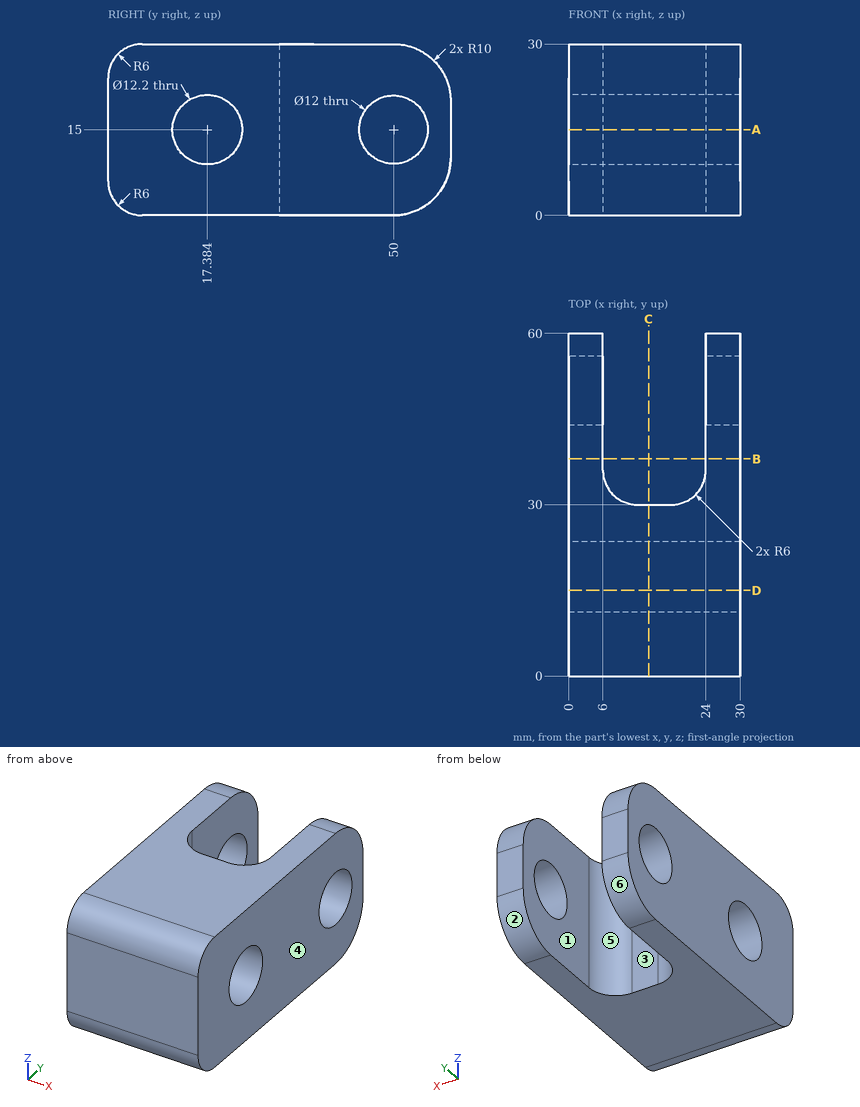
Answer from the drawing. Dimensions are ordinates in mm from the lowest x, y and z of the part. A direction names the side the tool comes from. Coordinates: 2 decimals unless noted, no trailing zeros. Loops run counter-clockwise (first coordinate to the right, second up) from the corner with the lowest first, then second, coordinate; pieces in that order, holes last. Notation, with made-up numbers: (-22, 42) -> (35, 42) arc R18 ccw to (35, 46) -> close; hole circle Ø1 at (-16.75, 8.5). An arc over 180 degrees is marked (long way). Return JSON: item names as keys, results as strings.
Item 1: Find section C-C (x = 14). Determine the outline of the cut face in (y, z).
Answers:
{"outline": "(0, 6) arc R6 ccw to (6, 0) -> (30, 0) -> (30, 30) -> (6, 30) arc R6 ccw to (0, 24) -> close; hole circle Ø12.2 at (17.38, 15)"}
Item 2: For the marked faces 1 and 2, determine the directions among +Z, -Z, +X, -X, +Y, -Y from which every point of the face is accessible in a straight line to the end or side of a thin tool.
Answers:
{"face 1": "+Z, -Z, +Y", "face 2": "-Z, +X, -X, +Y"}
Item 3: Find section D-D (y = 15). Determine the outline of the cut face in (x, z) (1 decimal).
Answers:
{"outline": "(0, 0) -> (30, 0) -> (30, 9.4) -> (0, 9.4) -> close; (0, 20.6) -> (30, 20.6) -> (30, 30) -> (0, 30) -> close"}
Item 4: Find section B-B (y = 38). Determine the outline of the cut face in (x, z), plus the area to 3 significant figures.
Answers:
{"outline": "(0, 0) -> (6, 0) -> (6, 30) -> (0, 30) -> close; (24, 0) -> (30, 0) -> (30, 30) -> (24, 30) -> close", "area": "360 mm2"}
Item 5: Find section A-A (z = 15). Determine the outline of the cut face in (x, y).
Answers:
{"outline": "(0, 0) -> (30, 0) -> (30, 11.28) -> (0, 11.28) -> close; (0, 23.48) -> (30, 23.48) -> (30, 44) -> (24, 44) -> (24, 36) arc R6 cw to (18, 30) -> (12, 30) arc R6 cw to (6, 36) -> (6, 44) -> (0, 44) -> close; (0, 56) -> (6, 56) -> (6, 60) -> (0, 60) -> close; (24, 56) -> (30, 56) -> (30, 60) -> (24, 60) -> close"}
Item 6: Flat-ended cylindrical pins translate along their axes: P1, Ø7, axis at y = 50, z = 15, coming from the -X side; P2, Ø6.5, axis at x = 15.5, z = 16, coming from the +Y side. Find the tip coordinate at first contact, or state that the pin passes through.
Answers:
{"P1": "passes through", "P2": "stops at y = 30.05"}
Item 7: For a pull along X with two mould halves and no side action, classify the marked faces 3, 4, 5 and 6 as +X half, -X half, draft (parallel to the pull), parting line (faces both ways), or undercut.
Answers:
{"face 3": "undercut", "face 4": "+X half", "face 5": "undercut", "face 6": "draft"}
Item 8: Find the intervals of material crossed by probe 1 along Z at (x, y) = (2.2, 50); probe 2 along X at (y, z) = (41, 8.75); probe 3 along Y at (x, z) = (16.75, 5.75) (1 decimal), in increasing order.
Answers:
{"probe 1": "z = 0 to 9, 21 to 30", "probe 2": "x = 0 to 6, 24 to 30", "probe 3": "y = 0 to 30"}
